Geometry: see drawing. Coordinates: mm, zero at the bounding-box minimum. A direction names the side the tool comes from. Coordinates: 2 decimals unless noted, no trailing zeros. Loops run counter-clockwise (first coordinate to the right, second up) from the corner with the lowest first, then second, coordinate; pieces in that order, holes last. Notation, with made-up numbers: (26.5, 36.5) - (53.5, 36.5) arc R17 ccw to (53.5, 41.5) - close; hole circle Ø6 at (86.25, 79). An arc over 180 degrees is marked (long way). Answer in a Markdown table with one row per item.
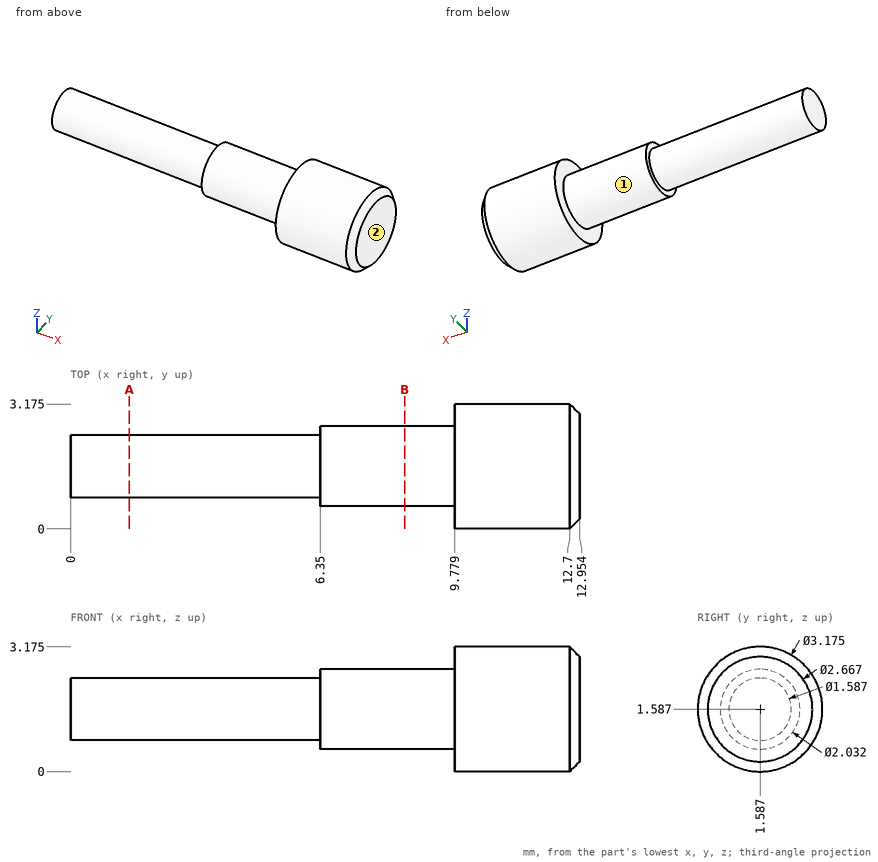
(1) First-contact query: pin 1 Ø1 at (y, z) = (0.5, 0.5) entering from +X; pin 2 Ø1 at (x, y) = (6, 1) entering from -Z. Flat tips, straight axial feed; report the tip coordinate or a pass-through.
Verdict:
| item | result |
|---|---|
| pin 1 | stops at x = 12.95 |
| pin 2 | stops at z = 0.6 |
(2) Cut plane A-A on x = 1.5. Output: boundary loops of the cut face in (y, z).
Verdict:
| item | result |
|---|---|
| outline | circle Ø1.59 at (1.59, 1.59) |
(3) Ray query, probe 1 along Z at (x, y) = (6.5, 1.6); probe 2 along X at (y, z) = (2.45, 0.85) (1 decimal). Return the intervals inside material, ascending.
Verdict:
| item | result |
|---|---|
| probe 1 | z = 0.57 to 2.6 |
| probe 2 | x = 9.8 to 13 |
(4) Cut plane B-B on x = 8.5. Output: boundary loops of the cut face in (y, z) (1 decimal).
Verdict:
| item | result |
|---|---|
| outline | circle Ø2 at (1.6, 1.6) |
(5) Access query for the marked faces 1 and 2. Directions: +Z, -Z, +X, -X, +Y, -Y. A direction counts if a zero-diameter tool reaches every point of the face in a straight line with its end or side. Return the directions, or none.
Verdict:
| item | result |
|---|---|
| face 1 | -X |
| face 2 | +Z, -Z, +X, +Y, -Y |
